CAD build for the part. Positions are in the model's coordinates, mm. Face numbers are marked on the shaded views. Coordinates: 2 decimals unless noted, no trailing zeros. Order: outer loops, then holes, each group sorted by start corner. A loop starts at its lowest first (then second) coordinate and runs counter-clockwise, first axis right, second up. Notation, with made-up numbers: (-9, 87.5) - (25, 87.5) arc R21 ccw to (25, 102.5) - close; hole circle Ø11 at (-36, 58.5). An arc over 180 degrees is marked (long way). Use one line per item in the form item = value.
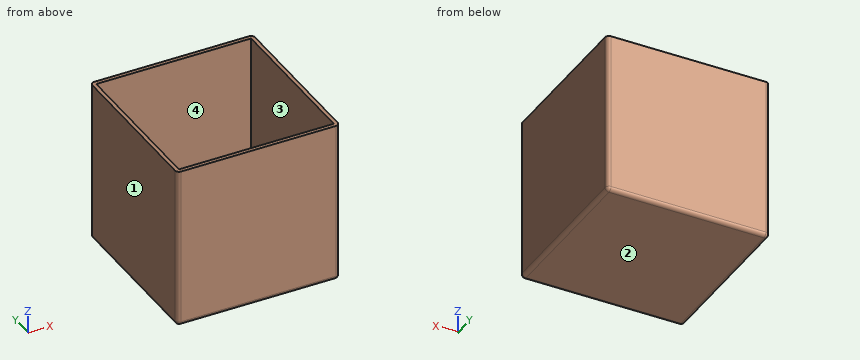
```python
from build123d import *

# Parameters (mm, degrees)
F0_W     = 50
F0_H     = 50
F1_DEPTH = 50
F2_T     = -1.2
F3_R     = 1.2
F4_R     = 1.2


with BuildPart() as f1:
    # F0 (on Top) → F1 (new body)
    with BuildSketch(Plane.XY):
        with Locations((-25, 25)):
            Rectangle(F0_W, F0_H)
    extrude(amount=F1_DEPTH)

    # F2
    f2_openings = [f1.faces().sort_by_distance(p)[0] for p in [
        (-25, 25, 50),
    ]]
    offset(amount=F2_T, openings=f2_openings)

    # F3
    f3_edges = [f1.edges().sort_by_distance(p)[0] for p in [
        (-50, 50, 25),
        (-50, 0, 25),
        (0, 0, 25),
        (0, 50, 25),
    ]]
    fillet(f3_edges, radius=F3_R)

    # F4
    f4_edges = [f1.edges().sort_by_distance(p)[0] for p in [
        (-25, 50, 0),
        (-50, 25, 0),
        (0, 25, 0),
        (-25, 0, 0),
    ]]
    fillet(f4_edges, radius=F4_R)


solid = f1.part
```
Item 1: Cut at A-A, the plane x = -38.5. Write the cut outline in (y, z).
Derived:
outline = (0, 1.2) arc R1.2 ccw to (1.2, 0) - (48.8, 0) arc R1.2 ccw to (50, 1.2) - (50, 50) - (48.8, 50) - (48.8, 1.2) - (1.2, 1.2) - (1.2, 50) - (0, 50) - close
Item 2: Cut at C-C, the plane y = 31.5. Write the cut outline in (x, z).
Derived:
outline = (-50, 1.2) arc R1.2 ccw to (-48.8, 0) - (-1.2, 0) arc R1.2 ccw to (0, 1.2) - (0, 50) - (-1.2, 50) - (-1.2, 1.2) - (-48.8, 1.2) - (-48.8, 50) - (-50, 50) - close
Item 3: Drill centre lines: line 1 (Y direction, x = -47.5, z = 40); line 2 (X direction, y = 37, z = 44); line 3 (Z direction, x = -2.5, y = 19.5). Where is each one in solid material? Low to high. Write a range as [from, to].
Derived:
line_1 = [0, 1.2], [48.8, 50]
line_2 = [-50, -48.8], [-1.2, 0]
line_3 = [0, 1.2]
Item 4: Drop a flat-ended pin along its axis: pin 1 (14.5 mm diameter, centred on x = -25, y = 18, fed in from +Z). Give the stop position or say it passes through.
Derived:
pin_1 = 1.2
Item 5: Two-plate mould, pull along X, no slides. Class the marked faces 1, 2, 3 and 4: +X half, -X half, draft (parallel to the pull), parting line (faces both ways), or undercut.
Derived:
face_1 = -X half
face_2 = draft
face_3 = undercut
face_4 = undercut
Item 6: Cut at B-B, the plane z = 41. Write the cut outline in (x, y).
Derived:
outline = (-50, 1.2) arc R1.2 ccw to (-48.8, 0) - (-1.2, 0) arc R1.2 ccw to (0, 1.2) - (0, 48.8) arc R1.2 ccw to (-1.2, 50) - (-48.8, 50) arc R1.2 ccw to (-50, 48.8) - close; hole (-48.8, 1.2) - (-1.2, 1.2) - (-1.2, 48.8) - (-48.8, 48.8) - close
